Work out the finished part from the listing and answer in its coordinate system (mm). A direction names the side the tool comes from. Coordinates: 2 decimals unless noted, no trailing zeros. Order: outer loops, then holes, each group sorted by start corner. A loop starts at its lowest first (then second) coordinate and runs counter-clockwise, first axis right, second up. Notation, with made-up numbers: M -19.75,55 L -6.75,55 A21 ccw -6.75,63 Z; hole C -14.5,55 d11. An arc over 180 degrees is marked long. Write item = value, one per line. Start each with the question number.
Q1. A tool of negligible diameter and unlimited length cuts with its end or side. For faces 1 (the flat face through (2, 2, 0)), 2 (the flat face through (0, -2.5, 3)), 3 (the flat face through (2.174, -1.234, 2.849)), from which of +Z, -Z, +X, -X, +Y, -Y can it reach the whole face along a straight path? Write none if from no direction.
Q2. Each of these flat-tipped pins is pushed along its axis until it touches: P1, Ø1.5, axis at x = 0, z = -22, coming from the -Y side; P2, Ø3, axis at x = -0.5, z = 3.5, coming from the +Y side; P3, Ø3, axis at x = -3, z = -21.5, coming from the -Y side. Where does it stop, or does it pass through?
Q3. Find section B-B on z = -9.75. Give the vertices of the cut face in (x, y).
Q4. Straight lines are drawn through the part: line 1 along Y through (x, z) = (0.75, 2.75); line 2 along X through (y, z) = (1.25, -6.5); line 3 along X through (y, z) = (1.5, -17.75). For each, find the intervals that lie inside material, in ascending order.
Q5. Find section A-A on x = 0. Give the vertices of the cut face in (y, z), and give its area (3 significant figures).
Autodesk Inventor part; units mm, degrees
ref_plane "YZ Plane" through (0, 0, 0) normal (1, 0, 0) x (0, 1, 0)
ref_plane "XZ Plane" through (0, 0, 0) normal (0, 1, 0) x (-1, 0, 0)
ref_plane "XY Plane" through (0, 0, 0) normal (0, 0, 1) x (1, 0, 0)
sketch "草图1" plane through (0, 0, 0) normal (0, 0, 1) x (1, 0, 0)
  circle A0 centre (0, 0) radius 4
  dimension "d0" = 8
extrude "拉伸1" add sketch "草图1" along normal blind 1
sketch "草图2" plane through (0, 0, 1) normal (0, 0, 1) x (1, 0, 0)
  line L0 (1.4434, -2.5) -> (-1.4434, -2.5)
  line L1 (-1.4434, -2.5) -> (-2.8868, 0)
  line L2 (-2.8868, 0) -> (-1.4434, 2.5)
  line L3 (-1.4434, 2.5) -> (1.4434, 2.5)
  line L4 (1.4434, 2.5) -> (2.8868, 0)
  line L5 (2.8868, 0) -> (1.4434, -2.5)
  line L6 (0, 0) -> (0, 1.5067)
  point P0 (0, 2.5)
  dimension "d3" = 1.5067
  dimension "d4" = 5
extrude "拉伸2" add sketch "草图2" along normal blind 4
sketch "草图3" plane through (0, 0, 0) normal (0, 0, -1) x (-1, 0, 0)
  circle A0 centre (0, 0) radius 2.5
  dimension "d7" = 5
extrude "拉伸3" add sketch "草图3" along normal blind 25
thread "螺纹1"
chamfer "倒角1" distance 0.25 angle 45 1 edges at (2.5, 0, -25)
fillet "圆角1" radius 0.25 13 edges at (-4, 0, 1) (0, 2.5, 5) (2.1651, 1.25, 5) (2.1651, -1.25, 5) (0, -2.5, 5) (-2.1651, -1.25, 5) (-2.1651, 1.25, 5) (1.4434, 2.5, 3) (2.8868, 0, 3) (1.4434, -2.5, 3) (-1.4434, -2.5, 3) (-2.8868, 0, 3) (-1.4434, 2.5, 3)
properties part number "刀夹片紧固螺丝"
Findings below:
q1.face_1 = -Z
q1.face_2 = +Z, +X, -X, -Y
q1.face_3 = +Z, +X, -Y
q2.P1 = -2.5
q2.P2 = 2.5
q2.P3 = -2
q3.outline = C 0,0 d5
q4.line_1 = -2.5 to 2.5
q4.line_2 = -2.17 to 2.17
q4.line_3 = -2 to 2
q5.outline = M -4,0 L -2.5,0 L -2.5,-24.75 L -2.25,-25 L 2.25,-25 L 2.5,-24.75 L 2.5,0 L 4,0 L 4,0.75 A0.25 ccw 3.75,1 L 2.5,1 L 2.5,4.75 A0.25 ccw 2.25,5 L -2.25,5 A0.25 ccw -2.5,4.75 L -2.5,1 L -3.75,1 A0.25 ccw -4,0.75 Z
q5.area = 153 mm^2
